The model under review builds one solid part; all positions refer to its coordinate system, in mm. A direction names the side the tool comes from. Round coordinates to 2 decimals unless told otherwise and drop trailing zeros. Write each loop counter-clockwise with the first axis right and the second up, starting at its lowest first coordinate (ties: lowest second). Pieces come first, ordered by that corner, then holes. Notation, with made-up numbers: (-12.75, -39.75) -> (-5.75, -39.75) arc R21 ccw to (-5.75, -22.75) -> close; hole circle Ø11 at (23.5, 80). An arc over 180 degrees is marked (long way). Return JSON: item names as keys, results as strings. Group by question number.
1. Tool access review of faces 1 (the flat face through (-17.78, -128, 3)), 2 (the flat face through (17.78, -130, 3)), 3 (the flat face through (-19.05, 32, 3)): name each direction out of +Z, -Z, +X, -X, +Y, -Y from which nothing blocks a thin tool from reaching the whole face with its end or side.
2. Take a section at A-A, the plane x = 0. Write out the cut boundary in (y, z) (3 decimals), then the cut area to 3 significant figures.
3. Clearance check with flat-ended pins moving along their axes: P1, Ø2, axis at y = 31.5, z = 4.5, coming from the +X side; P2, Ø2, axis at y = -58.5, z = 5, coming from the -X side; P3, Ø11.5, axis at x = -31.43, y = 31.43, coming from the -Z side; P4, Ø2, axis at y = -114, z = 2.5, coming from the -X side. State where each tip first meets the part, or that it passes through.
4. Take a section at B-B, the plane y = 0. Write out the cut boundary in (x, z) (3 decimals), then the cut area to 3 significant figures.
5. Mouldability with a two-part tool opening along Y and no side actions: class faces 4 (the cylindrical face through (-25.374, 33.338, 3.444)), 5 (the cylindrical face through (-38.393, 1.907, 3.444)), 6 (the cylindrical face through (-57.075, -2.931, 3.444)), 7 (the cylindrical face through (-18.885, -55.158, 3.444)) as pulls with the +Y half, pulls with the -Y half, needs draft (parallel to the pull), parting line crosses it, or undercut.
6. For line 1 along X through (y, z) = (-3, 3); line 2 along X through (y, z) = (-33.5, 0.5); line 3 along Y through (x, z) = (25, 5.25), list the stretches that pass through material, from the lowest coordinate up. Write a range as from..to.
7. Take a section at D-D, the plane y = -143. Write out the cut boundary in (x, z) (3 decimals).
8. Take a section at C-C, the plane x = 43.5. Write out the cut boundary in (y, z) (3 decimals), then the cut area to 3 significant figures.
from build123d import *

# Parameters (mm, degrees)
F0_R     = 6.35
F1_DEPTH = 6.985


with BuildPart() as f1:
    # F0 (on Top) → F1 (new body)
    with BuildSketch(Plane.XY):
        with BuildLine():
            ThreePointArc((-19.05, 43.994091), (-22.225, 49.493352), (-28.575, 49.493352))
            ThreePointArc((-28.575, 49.493352), (-57.022152, -3.820554), (-21.717, -52.862978))
            ThreePointArc((-21.717, -52.862978), (-18.855294, -55.201112), (-17.78, -58.736642))
            Line((-17.78, -58.736642), (-17.78, -198.436642))
            ThreePointArc((-17.78, -198.436642), (-15.920128, -202.92677), (-11.43, -204.786642))
            Line((-11.43, -204.786642), (11.43, -204.786642))
            ThreePointArc((11.43, -204.786642), (15.920128, -202.92677), (17.78, -198.436642))
            Line((17.78, -198.436642), (17.78, -58.736642))
            ThreePointArc((17.78, -58.736642), (18.855294, -55.201112), (21.717, -52.862978))
            ThreePointArc((21.717, -52.862978), (57.022152, -3.820554), (28.575, 49.493352))
            ThreePointArc((28.575, 49.493352), (22.225, 49.493352), (19.05, 43.994091))
            Line((19.05, 43.994091), (19.05, 21.298547))
            ThreePointArc((19.05, 21.298547), (0, -28.575), (-19.05, 21.298547))
            Line((-19.05, 21.298547), (-19.05, 43.994091))
        make_face()
        with Locations((-31.430896, -31.430896)):
            Circle(F0_R, mode=Mode.SUBTRACT)
        with Locations((0, -44.45)):
            Circle(F0_R, mode=Mode.SUBTRACT)
        with Locations((-44.45, 0)):
            Circle(F0_R, mode=Mode.SUBTRACT)
        with Locations((-31.430896, 31.430896)):
            Circle(F0_R, mode=Mode.SUBTRACT)
        with Locations((31.430896, -31.430896)):
            Circle(F0_R, mode=Mode.SUBTRACT)
        with Locations((44.45, 0)):
            Circle(F0_R, mode=Mode.SUBTRACT)
        with Locations((31.430896, 31.430896)):
            Circle(F0_R, mode=Mode.SUBTRACT)
    extrude(amount=F1_DEPTH)


solid = f1.part
Output:
{
 "1": {"face 1": "+Z, -Z, -X, -Y", "face 2": "+Z, -Z, +X, -Y", "face 3": "+Z, -Z, +Y"},
 "2": {"outline": "(-204.787, 0) -> (-50.8, 0) -> (-50.8, 6.985) -> (-204.787, 6.985) -> close; (-38.1, 0) -> (-28.575, 0) -> (-28.575, 6.985) -> (-38.1, 6.985) -> close", "area": "1,140 mm^2"},
 "3": {"P1": "stops at x = 48.33", "P2": "stops at x = -17.9", "P3": "passes through", "P4": "stops at x = -17.78"},
 "4": {"outline": "(-57.15, 0) -> (-50.8, 0) -> (-50.8, 6.985) -> (-57.15, 6.985) -> close; (-38.1, 0) -> (-28.575, 0) -> (-28.575, 6.985) -> (-38.1, 6.985) -> close; (28.575, 0) -> (38.1, 0) -> (38.1, 6.985) -> (28.575, 6.985) -> close; (50.8, 0) -> (57.15, 0) -> (57.15, 6.985) -> (50.8, 6.985) -> close", "area": "222 mm^2"},
 "5": {"face 4": "undercut", "face 5": "undercut", "face 6": "parting line crosses it", "face 7": "pulls with the -Y half"},
 "6": {"line 1": "x = -57.07..-50.05, -38.85..-28.42, 28.42..38.85, 50.05..57.07", "line 2": "x = -46.3..-37.43, -25.43..25.43, 37.43..46.3", "line 3": "y = -51.39..-13.84, 13.84..50.33"},
 "7": {"outline": "(-17.78, 0) -> (17.78, 0) -> (17.78, 6.985) -> (-17.78, 6.985) -> close"},
 "8": {"outline": "(-37.066, 0) -> (-6.279, 0) -> (-6.279, 6.985) -> (-37.066, 6.985) -> close; (6.279, 0) -> (37.066, 0) -> (37.066, 6.985) -> (6.279, 6.985) -> close", "area": "430 mm^2"}
}
